Could you check a few things on this model? Use its own coordinates, in mm. A direction names the side the tool comes from. Give positions to 0.01 mm unless a question says otherwise; leave off trailing zeros. Write each loop counter-clockwise with the first axis right and the second up, starting at its lowest first coordinate (ties: lowest second). Pieces come first, ordered by that corner, then holes. Notation, with made-up numbers: (82, 52.25) - (101, 52.25) arc R11 ccw to (101, 56.25) - close; hole circle Ø1 at (-23.75, 59.5). An arc over 180 degrees is marked (long way). Answer in a Markdown table with one row per item.
from build123d import *

# Parameters (mm, degrees)
F0_R     = 19.05
F1_DEPTH = 76.2
F2_W     = 152.4
F2_H     = 50.8
F2_R     = 19.05
F3_DEPTH = 12.7
F4_W     = 12.7
F4_H     = 50.8
F5_DEPTH = 50.8
F6_R     = 12.7
F7_DEPTH = 304.8


with BuildPart() as f1:
    # F0 (on Top) → F1 (new body)
    with BuildSketch(Plane.XY):
        Circle(F0_R)
    extrude(amount=F1_DEPTH)

    # F2 (on face) → F3 (join)
    with BuildSketch(Plane.XY.offset(76.2)):
        Rectangle(F2_W, F2_H)
        Circle(F2_R, mode=Mode.SUBTRACT)
        Circle(F2_R)
    extrude(amount=F3_DEPTH)

    # F4 (on face) → F5 (join)
    with BuildSketch(Plane.XY.offset(88.9)):
        with Locations((-69.85, 0)):
            Rectangle(F4_W, F4_H)
        with Locations((69.85, 0)):
            Rectangle(F4_W, F4_H)
    extrude(amount=F5_DEPTH)

    # F6 (on face) → F7 (cut)
    with BuildSketch(Plane(origin=(-76.2, 0, 0), x_dir=(0, -1, 0), z_dir=(-1, 0, 0))):
        with Locations((0, 120.65)):
            Circle(F6_R)
    extrude(amount=-F7_DEPTH, mode=Mode.SUBTRACT)


solid = f1.part
1) Imagine slicing it at B-B (z = 120.65). List the corners of the cut face in (x, y) for me, then the cut area to 3 significant figures.
Check values:
| item | result |
|---|---|
| outline | (-76.2, -25.4) - (-63.5, -25.4) - (-63.5, -12.7) - (-76.2, -12.7) - close; (-76.2, 12.7) - (-63.5, 12.7) - (-63.5, 25.4) - (-76.2, 25.4) - close; (63.5, -25.4) - (76.2, -25.4) - (76.2, -12.7) - (63.5, -12.7) - close; (63.5, 12.7) - (76.2, 12.7) - (76.2, 25.4) - (63.5, 25.4) - close |
| area | 645 mm2 |
2) Imagine slicing it at D-D (y = 22.5). List the corners of the cut face in (x, z) for me.
Check values:
| item | result |
|---|---|
| outline | (-76.2, 76.2) - (76.2, 76.2) - (76.2, 139.7) - (63.5, 139.7) - (63.5, 88.9) - (-63.5, 88.9) - (-63.5, 139.7) - (-76.2, 139.7) - close |
3) If I drill on line 1 (Y direction, x = -70, z = 120); line 2 (X direction, y = 13.5, z = 115); line 3 (Z direction, x = 2, y = 20.5), over which ranges is the centre line in solid material (lowest first)?
Check values:
| item | result |
|---|---|
| line 1 | y = -25.4 to -12.68, 12.68 to 25.4 |
| line 2 | x = -76.2 to -63.5, 63.5 to 76.2 |
| line 3 | z = 76.2 to 88.9 |
4) Imagine slicing it at C-C (x = 0). List the corners of the cut face in (y, z) for me, then the cut area to 3 significant figures.
Check values:
| item | result |
|---|---|
| outline | (-25.4, 76.2) - (-19.05, 76.2) - (-19.05, 0) - (19.05, 0) - (19.05, 76.2) - (25.4, 76.2) - (25.4, 88.9) - (-25.4, 88.9) - close |
| area | 3,550 mm2 |
5) On a 3-axis mill with a long thin cutter (end or side, diameter ignored), from which of +Z, -Z, +X, -X, +Y, -Y can I reach the whole of each face in a straight line? I mean faces 1 (the face through (-76.2, -0.4, 107.5)), 2 (the face through (-15.12, -11.59, 37.57)), 3 (the face through (-63.5, 5, 108)). Say none if no direction works.
Check values:
| item | result |
|---|---|
| face 1 | +Z, -Z, -X, +Y, -Y |
| face 2 | -Z |
| face 3 | +Z, +Y, -Y |
6) Imagine slicing it at A-A (y = 0). List the corners of the cut face in (x, z) for me.
Check values:
| item | result |
|---|---|
| outline | (-76.2, 76.2) - (-19.05, 76.2) - (-19.05, 0) - (19.05, 0) - (19.05, 76.2) - (76.2, 76.2) - (76.2, 107.95) - (63.5, 107.95) - (63.5, 88.9) - (-63.5, 88.9) - (-63.5, 107.95) - (-76.2, 107.95) - close; (-76.2, 133.35) - (-63.5, 133.35) - (-63.5, 139.7) - (-76.2, 139.7) - close; (63.5, 133.35) - (76.2, 133.35) - (76.2, 139.7) - (63.5, 139.7) - close |
7) We'd pull the mould along Z, two halves only. Please class faces 4 (the face through (-69.939, -5.86, 109.383)), 5 (the face through (63.5, 5, 108)), 6 (the face through (70, 0, 139.7)): +Z half, -Z half, draft (parallel to the pull), parting line (faces both ways), or undercut.
Check values:
| item | result |
|---|---|
| face 4 | undercut |
| face 5 | draft |
| face 6 | +Z half |
8) Will these pins go through, and if not, where does the flat tip stop? P1, Ø5, axis at x = -38.5, y = -5.5, coming from the -Z side; P2, Ø3, axis at x = -28.5, y = -14.5, coming from the +Z side; P3, Ø2, axis at y = 8, z = 58, coming from the +X side.
Check values:
| item | result |
|---|---|
| P1 | stops at z = 76.2 |
| P2 | stops at z = 88.9 |
| P3 | stops at x = 17.72 |
